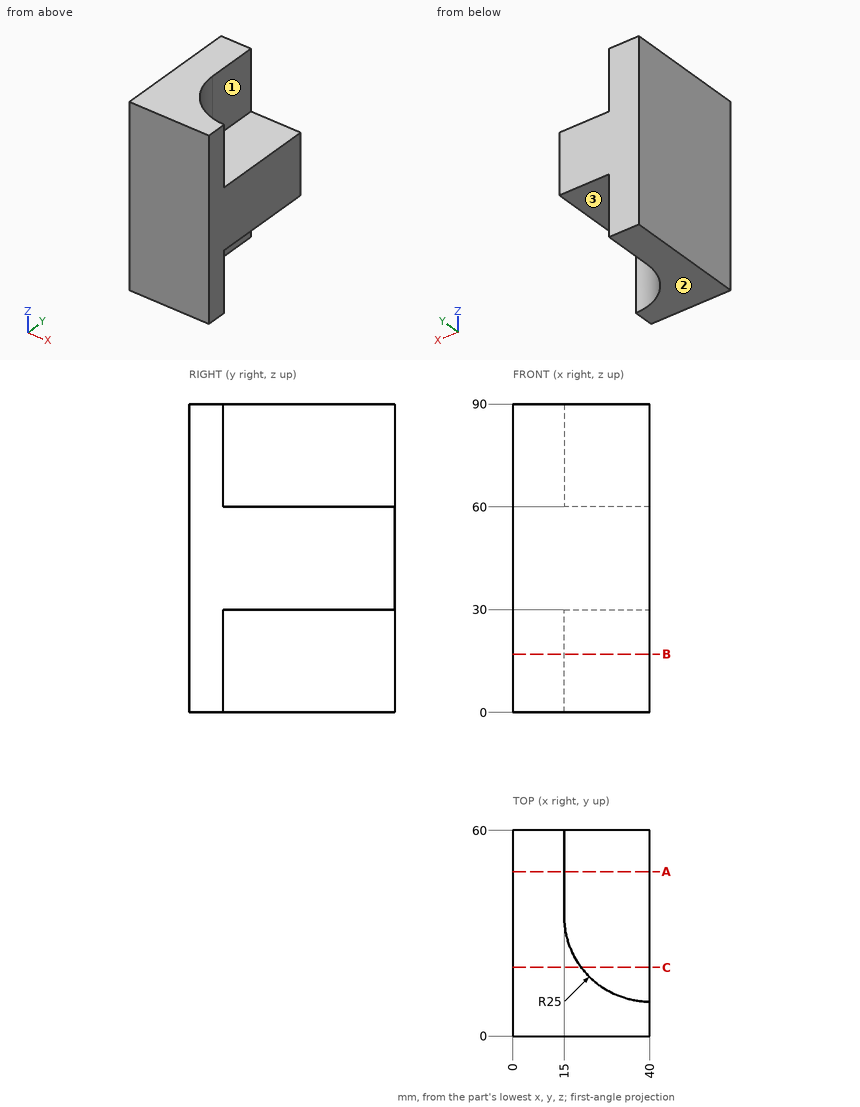
Job drawing, mm, ordinate dimensions from the low corner. One solid piece. A direction names the side the tool comes from. Give positions to 0.01 mm unless a question says otherwise; leave off trailing zeros. Loops run counter-clockwise (first coordinate to the right, second up) from the corner with the lowest first, then second, coordinate; pieces in that order, holes last. Notation, with made-up numbers: M 84.5,-26 L 109.5,-26 A21 ccw 109.5,-3 Z; hole C 57,-10 d8. An arc over 180 degrees is marked long. Answer in a Markdown table with one row per item. Add a question column.
Item 1: Band-saw the part on C-C on y = 20. Give the cut face in (x, z).
Item 2: Band-saw the part on A-A on y = 48. Give the cut face in (x, z), then the cut area to 3 significant figures.
Item 3: Drop flat-ended pins along their axis: P1, Ø12.5, axis at y = 45.5, z = 69.5, coming from the +X side; P2, Ø5, axis at y = 33, z = 56.5, coming from the -X side; P3, Ø6, axis at x = 35, y = 32.5, coming from the +Z side; P4, Ø7.5, axis at x = 24.5, y = 47, coming from the -Z side. Give the stop position or say it passes through.
Item 4: Band-saw the part on B-B on z = 17. Give the cut face in (x, y).
Item 5: Tool access for the marked faces 1, 2 and 3: list every direction of +Z, -Z, +X, -X, +Y, -Y with a clear straight run to the whole face (end or side of a thin tool).
Item 6: Probe probe 1 along X at (y, z) = (46, 10); probe 2 along Z at (x, y) = (32, 35); probe 3 along X at (y, z) = (18, 28). List the from-to ranges inside material, lowest first.
Reply:
| question | item | result |
|---|---|---|
| 1 | outline | M 0,0 L 20,0 L 20,30 L 40,30 L 40,60 L 20,60 L 20,90 L 0,90 Z |
| 2 | outline | M 0,0 L 15,0 L 15,30 L 40,30 L 40,60 L 15,60 L 15,90 L 0,90 Z |
| 2 | area | 2,100 mm^2 |
| 3 | P1 | stops at x = 15 |
| 3 | P2 | stops at x = 0 |
| 3 | P3 | stops at z = 60 |
| 3 | P4 | stops at z = 30 |
| 4 | outline | M 0,0 L 40,0 L 40,10 A25 cw 15,35 L 15,60 L 0,60 Z |
| 5 | face 1 | +Z, +X, +Y |
| 5 | face 2 | -Z, +X, -X, +Y, -Y |
| 5 | face 3 | -Z, +X, +Y |
| 6 | probe 1 | x = 0 to 15 |
| 6 | probe 2 | z = 30 to 60 |
| 6 | probe 3 | x = 0 to 21.67 |
